Part model, mm, in its own coordinate system. Coordinates: 2 decimals unless noted, no trailing zeros. Loops run counter-clockwise (first coordinate to the right, second up) from the corner with the lowest first, then second, coordinate; pieces in that order, holes last.
```python
from build123d import *

# Parameters (mm, degrees)
ESQUISSE1_W             = 350
ESQUISSE1_H             = 360
ESQUISSE1_R             = 3.175
ESQUISSE1_W_2           = 310
ESQUISSE1_H_2           = 320
BOSS_EXTRU_2_DEPTH      = 23.5
ENL_V_START             = 2
ESQUISSE1_4_W           = 346
ESQUISSE1_4_H           = 356
ENL_V_MAT_EXTRU_1_DEPTH = 19.5


with BuildPart() as part:
    # Esquisse1 → Boss.-Extru.2 (new body)
    with BuildSketch(Plane(origin=(0, 0, 0), x_dir=(1, 0, 0), z_dir=(0, 1, 0))):
        with Locations((175, 180)):
            Rectangle(ESQUISSE1_W, ESQUISSE1_H)
        with Locations((10, 10)):
            Circle(ESQUISSE1_R, mode=Mode.SUBTRACT)
        with Locations((175, 10)):
            Circle(ESQUISSE1_R, mode=Mode.SUBTRACT)
        with Locations((340, 10)):
            Circle(ESQUISSE1_R, mode=Mode.SUBTRACT)
        with Locations((340, 180)):
            Circle(ESQUISSE1_R, mode=Mode.SUBTRACT)
        with Locations((10, 180)):
            Circle(ESQUISSE1_R, mode=Mode.SUBTRACT)
        with Locations((340, 350)):
            Circle(ESQUISSE1_R, mode=Mode.SUBTRACT)
        with Locations((175, 350)):
            Circle(ESQUISSE1_R, mode=Mode.SUBTRACT)
        with Locations((10, 350)):
            Circle(ESQUISSE1_R, mode=Mode.SUBTRACT)
        with Locations((175, 180)):
            Rectangle(ESQUISSE1_W_2, ESQUISSE1_H_2, mode=Mode.SUBTRACT)
    extrude(amount=BOSS_EXTRU_2_DEPTH)

    # Esquisse1_4 → Enl_v. mat.-Extru.1 (cut)
    with BuildSketch(Plane(origin=(0, 0, 0), x_dir=(1, 0, 0), z_dir=(0, 1, 0)).offset(ENL_V_START)):
        with Locations((175, 180)):
            Rectangle(ESQUISSE1_4_W, ESQUISSE1_4_H)
    extrude(amount=ENL_V_MAT_EXTRU_1_DEPTH, mode=Mode.SUBTRACT)


solid = part.part
```
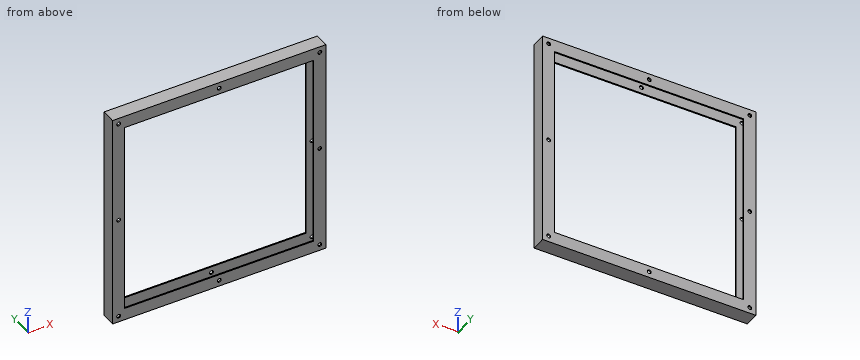
Q1. Saw through at B-B (z = -195.5). List the corners of the cut face in (x, y), plus the area to 3 significant figures.
Q2. Probe line 1 (X direction, y = 22.3, z = -350) (3 decimals); line 2 (Z direction, x = 10, y = 23) (3 decimals); line 3 (X direction, y = 1.3, z = -180) (3 decimals). List the from-to ranges inside material, lowest first.
Q3. Saw through at A-A (x = 61). List the corners of the cut face in (y, z).
Q4. Drop flat-ended pins along their axis: P1, Ø3, axis at y = 11.5, z = -322, coming from the -X side; P2, Ø5, axis at x = 10, z = -180, coming from the -Y side. Give the stop position or say it passes through.
Q5. Saw through at C-C (y = 8). List the corners of the cut face in (x, z).
Checked values:
1. outline: (0, 0) - (20, 0) - (20, 2) - (2, 2) - (2, 21.5) - (20, 21.5) - (20, 23.5) - (0, 23.5) - close; (330, 0) - (350, 0) - (350, 23.5) - (330, 23.5) - (330, 21.5) - (348, 21.5) - (348, 2) - (330, 2) - close
1. area: 238 mm2
2. line 1: x = 0 to 6.825, 13.175 to 171.825, 178.175 to 336.825, 343.175 to 350
2. line 2: z = -360 to -353.175, -346.825 to -183.175, -176.825 to -13.175, -6.825 to 0
2. line 3: x = 0 to 6.825, 13.175 to 20, 330 to 336.825, 343.175 to 350
3. outline: (0, -360) - (23.5, -360) - (23.5, -340) - (21.5, -340) - (21.5, -358) - (2, -358) - (2, -340) - (0, -340) - close; (0, -20) - (2, -20) - (2, -2) - (21.5, -2) - (21.5, -20) - (23.5, -20) - (23.5, 0) - (0, 0) - close
4. P1: stops at x = 0
4. P2: passes through
5. outline: (0, -360) - (350, -360) - (350, 0) - (0, 0) - close; hole (2, -358) - (348, -358) - (348, -2) - (2, -2) - close
